For this review, use the dimensioned drawing (mm, ordinates from the lowest corner) and the shaded views. A direction names the side the tool comes from. Round coordinates to 2 decimals unless told otherwise and drop trailing zeros. Write each loop counter-clockwise with the first axis right and the second up, starting at its lowest first coordinate (ties: lowest second). Pieces come first, ordered by that corner, then holes. Notation, with made-up numbers: (63.5, -5.5) - (73.5, -5.5) arc R25 cw to (73.5, 27.5) - close; hole circle Ø1 at (-13.75, 62). An arc over 180 degrees is marked (long way). Return JSON: item names as keys, results as strings.
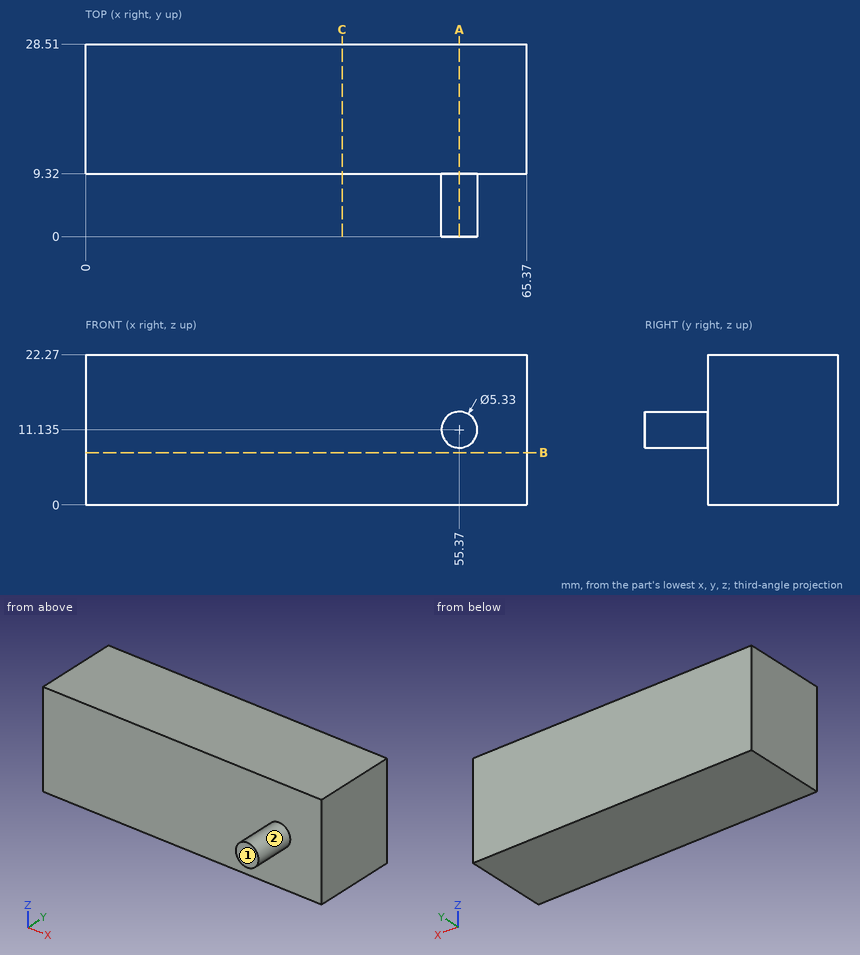
(1) For the marked faces 1 and 2, list the 3-axis set-ups (+Z, -Z, +X, -X, +Y, -Y) from which the entire face can be reached by the end or side of a thin tool; tool diameter is ignored.
Filled in:
{"face 1": "+Z, -Z, +X, -X, -Y", "face 2": "-Y"}
(2) Add section C-C (x = 38). Write out the cut boundary in (y, z).
Filled in:
{"outline": "(9.32, 0) - (28.51, 0) - (28.51, 22.27) - (9.32, 22.27) - close"}
(3) Add section B-B (z = 7.75). Write out the cut boundary in (x, y).
Filled in:
{"outline": "(0, 9.32) - (65.37, 9.32) - (65.37, 28.51) - (0, 28.51) - close"}
(4) Wall thickness on line 1 (X direction, y = 5.5, z = 11.25); line 2 (Y direction, x = 45, z = 7.75): over which ranges is each line inside the solid? List them lowest first.
Filled in:
{"line 1": "x = 52.71 to 58.03", "line 2": "y = 9.32 to 28.51"}
(5) Clearance check with flat-ended pins moving along their axes: pin 1 Ø2 at (x, z) = (44, 6.5) entering from -Y; pin 2 Ø6 at (x, y) = (52, 5) entering from +Z. State where each tip first meets the part, or that it passes through.
Filled in:
{"pin 1": "stops at y = 9.32", "pin 2": "stops at z = 13.77"}
(6) Add section A-A (x = 55.37). Write out the cut boundary in (y, z), plus the area to 3 significant figures.
Filled in:
{"outline": "(0, 8.47) - (9.32, 8.47) - (9.32, 0) - (28.51, 0) - (28.51, 22.27) - (9.32, 22.27) - (9.32, 13.8) - (0, 13.8) - close", "area": "477 mm2"}
